Check sheet for the modelled part. Datum: model origin and axes. Units: mm. A direction names the side the tool comes from. Round coordinates to 2 decimals unless told otherwise and drop trailing zeros. Order: outer loops, then holes, each group sorted by start corner. A loop starts at its lowest first (then second) coordinate and runs counter-clockwise, first axis right, second up. Notation, with made-up numbers: M -33,27.25 L 23,27.25 A27 cw 23,55.25 Z; hole C 6.25,-33.5 d8. An arc over 180 degrees is marked long. One line per item, written item: value. Start each with the question number.
(1) Cross-section at D-D, the plane y = -18.5. Enter the section's corners in (x, z).
(2) Thickness scan on L1, parallel to Z at x = 0, y = -2.45; L2, parallel to Y at x = 0, z = 2.95; L3, parallel to Y at x = -6, z = 14. Record the ranges inside material, lowest first.
(3) Cross-section at A-A, the plane z = 18.5. Enter the section's corners in (x, y).
(4) Release check for a two-part mould opening along X. For faces 3 (the face through (0.769, -15.039, 4.146)), 4 (the face through (-13, -11, 11)), 5 (the face through (11, -25.8, 3.5)) record: released by +X, released by -X, zero draft, split by the parting line, or undercut.
(5) Cross-section at B-B, the plane x = 0. Enter the section's corners in (y, z), and give its area (3 significant figures).
(6) Depth check by flat-ended pin: pin 1 Ø5 at (x, z) = (-6, 7) entering from -Y (3 decimals); pin 2 Ø9 at (x, z) = (0, 18.5) entering from -Y; pin 3 Ø6 at (x, z) = (5, 15) entering from -Y. Enter the tip coordinate at first touch or a pass-through.
(7) Access from +Z, -Z, +X, -X, +Y, -Y to the whole of each face (thin tool, end or side, straight path). Record for faces 1 (the face through (-0.769, -4.146, 15.039)), 2 (the face through (-12, -10, 10)).
(8) Cross-section at C-C, the plane z = 3. Enter the section's corners in (x, y), and give its area (3 significant figures).
from build123d import *

# Parameters (mm, degrees)
SKETCH_W        = 30
SKETCH_H        = 30
PAD_DEPTH       = 30
FILLET_R        = 14
BOX_W           = 30
BOX_H           = 30
BOX_DEPTH       = 30
SKETCH001_R     = 3.4
POCKET_DEPTH    = 7
SKETCH002_R     = 3.4
POCKET001_DEPTH = 7
CHAMFER_SIZE    = 3
CHAMFER001_SIZE = 1
SKETCH003_W     = 3
SKETCH003_H     = 8
PAD001_DEPTH    = 8
POCKET002_DEPTH = 30.001


with BuildPart() as part:
    # Sketch → Pad (new body)
    with BuildSketch(Plane.XZ):
        with Locations((0, 15)):
            Rectangle(SKETCH_W, SKETCH_H)
    extrude(amount=PAD_DEPTH)

    # Fillet
    fillet_edges = [part.edges().sort_by_distance(p)[0] for p in [
        (15, -30, 15),
        (-15, -30, 15),
    ]]
    fillet(fillet_edges, radius=FILLET_R)

    # Box → Box (cut)
    with BuildSketch(Plane(origin=(-15, -7, 7), x_dir=(1, 0, 0), z_dir=(0, -1, 0))):
        with Locations((15, 15)):
            Rectangle(BOX_W, BOX_H)
    extrude(amount=BOX_DEPTH, mode=Mode.SUBTRACT)

    # Sketch001 (on Face6 of Box) → Pocket (cut)
    with BuildSketch(Plane(origin=(0, -7, 18.5), x_dir=(1, 0, 0), z_dir=(0, -1, 0))):
        Circle(SKETCH001_R)
    extrude(amount=-POCKET_DEPTH, mode=Mode.SUBTRACT)

    # Sketch002 (on Face5 of Pocket) → Pocket001 (cut)
    with BuildSketch(Plane(origin=(0, -18.5, 7), x_dir=(-1, 0, 0), z_dir=(0, 0, 1))):
        Circle(SKETCH002_R)
    extrude(amount=-POCKET001_DEPTH, mode=Mode.SUBTRACT)

    # Chamfer
    chamfer_edges = [part.edges().sort_by_distance(p)[0] for p in [
        (-3.4, -7, 18.5),
        (3.4, -18.5, 7),
    ]]
    chamfer(chamfer_edges, length=CHAMFER_SIZE)

    # Chamfer001
    chamfer001_edges = [part.edges().sort_by_distance(p)[0] for p in [
        (15, -3.5, 30),
        (-15, -3.5, 30),
    ]]
    chamfer(chamfer001_edges, length=CHAMFER001_SIZE)

    # Sketch003 (on Face1 of Chamfer001) → Pad001 (join)
    with BuildSketch(Plane(origin=(0, -7, 7), x_dir=(1, 0, 0), z_dir=(0, -1, 0))):
        with Locations((13.5, 4)):
            Rectangle(SKETCH003_W, SKETCH003_H)
        with Locations((-13.5, 4)):
            Rectangle(SKETCH003_W, SKETCH003_H)
    extrude(amount=PAD001_DEPTH)

    # Sketch004 (on Face22 of Pad001) → Pocket002 (cut, through all)
    with BuildSketch(Plane(origin=(15, -7, 7), x_dir=(0, 0, 1), z_dir=(1, 0, 0))):
        Polygon((0, 8), (8, 0), (8, 8), align=None)
    extrude(amount=-POCKET002_DEPTH, mode=Mode.SUBTRACT)


solid = part.part
Values found:
1. outline: M -14.77,0 L -3.4,0 L -3.4,4 L -6.4,7 L -14.77,7 Z; M 3.4,0 L 14.77,0 L 14.77,7 L 6.4,7 L 3.4,4 Z
2. L1: 0 to 15.1, 21.9 to 30
2. L2: -30 to -21.9, -15.1 to 0
2. L3: -7 to 0
3. outline: M -15,-7 L -6.4,-7 L -3.4,-4 L -3.4,0 L -15,0 Z; M 3.4,-4 L 6.4,-7 L 15,-7 L 15,0 L 3.4,0 Z
4. face 3: undercut
4. face 4: zero draft
4. face 5: released by +X
5. outline: M -30,0 L -21.9,0 L -21.9,4 L -24.9,7 L -30,7 Z; M -15.1,0 L 0,0 L 0,15.1 L -4,15.1 L -7,12.1 L -7,7 L -12.1,7 L -15.1,4 Z; M -7,24.9 L -4,21.9 L 0,21.9 L 0,30 L -7,30 Z
5. area: 258 mm^2
6. pin 1: y = -29.775
6. pin 2: y = -5.1
6. pin 3: y = -7
7. face 1: -Y
7. face 2: +Z, -Y
8. outline: M -15,-16 A14 ccw -1,-30 L 1,-30 A14 ccw 15,-16 L 15,0 L -15,0 Z; hole C 0,-18.5 d6.8
8. area: 780 mm^2
